The listing builds one solid part. Answer for the finished solid, in the listing's coordinates (mm). A direction names the side the tool comes from. Coordinates: 2 decimals unless noted, no trailing zeros. Write each loop counter-clockwise with the first axis right and the second up, starting at its lowest first coordinate (ties: lowest second). Pieces come first, ordered by that corner, then holes. Notation, with made-up numbers: M -8,-6 L 9,-6 A28 cw 9,22 Z; hole C 8,66.25 d3. An arc over 180 degrees is marked long. Answer as CSV lines item,"result". Start each with the question number.
```python
from build123d import *

# Parameters (mm, degrees)
F1_DEPTH       = 9.525
F2_D           = 5.5
F2_CBORE_D     = 9.75
F2_CBORE_DEPTH = 5
F3_R           = 5.08
F4_DEPTH       = 5
F5_D           = 5.5


# Not quite as in the source:
# - a feature names something its author has since deleted; it is built from what else it names


with BuildPart() as f1:
    # F0 (on Front) → F1 (new body)
    with BuildSketch(Plane.XZ):
        with BuildLine():
            Line((10, -40), (10, 0))
            ThreePointArc((10, 0), (7.0710678119, 7.0710678119), (0, 10))
            Line((0, 10), (-53.34, 10))
            ThreePointArc((-53.34, 10), (-62.826927837, 3.1619930765), (-59.3395200276, -8.0003599568))
            Line((-59.3395200276, -8.0003599568), (-5.9995200276, -48.0003599568))
            ThreePointArc((-5.9995200276, -48.0003599568), (4.4724042597, -48.9441377526), (10, -40))
        make_face()
        Polygon((-20.36, -4.1698729811), (-20.4062613559, -4.25), (-25.3137386441, -4.25), (-27.7674772881, 0), (-25.3137386441, 4.25), (-20.4062613559, 4.25), (-20.36, 4.1698729811), (-20.3137386441, 4.25), (-15.4062613559, 4.25), (-12.9525227119, 0), (-15.4062613559, -4.25), (-20.3137386441, -4.25), align=None, mode=Mode.SUBTRACT)
        Polygon((-25.3137386441, -4.25), (-20.4062613559, -4.25), (-20.36, -4.1698729811), (-22.7674772881, 0), (-20.36, 4.1698729811), (-20.4062613559, 4.25), (-25.3137386441, 4.25), (-27.7674772881, 0), align=None)
        Polygon((-17.9525227119, 0), (-20.36, -4.1698729811), (-20.3137386441, -4.25), (-15.4062613559, -4.25), (-12.9525227119, 0), (-15.4062613559, 4.25), (-20.3137386441, 4.25), (-20.36, 4.1698729811), align=None)
        Polygon((-22.7674772881, 0), (-20.36, -4.1698729811), (-17.9525227119, 0), (-20.36, 4.1698729811), align=None)
    extrude(amount=F1_DEPTH)

    # F2 (through all)
    with Locations(Plane(origin=(0, 0, 0), x_dir=(1, 0, 0), z_dir=(0, 1, 0))):
        with Locations((0, 0), (0, 40), (-53.34, 0)):
            CounterBoreHole(F2_D / 2, F2_CBORE_D / 2, F2_CBORE_DEPTH)

    # F3
    f3_edges = [f1.edges().sort_by_distance(p)[0] for p in [
        (-26.67, 0, 10),
    ]]
    fillet(f3_edges, radius=F3_R)

    # F0 (on Front) → F4 (cut)
    with BuildSketch(Plane.XZ):
        Polygon((-25.3137386441, -4.25), (-20.4062613559, -4.25), (-20.36, -4.1698729811), (-22.7674772881, 0), (-20.36, 4.1698729811), (-20.4062613559, 4.25), (-25.3137386441, 4.25), (-27.7674772881, 0), align=None)
        Polygon((-22.7674772881, 0), (-20.36, -4.1698729811), (-17.9525227119, 0), (-20.36, 4.1698729811), align=None)
        Polygon((-17.9525227119, 0), (-20.36, -4.1698729811), (-20.3137386441, -4.25), (-15.4062613559, -4.25), (-12.9525227119, 0), (-15.4062613559, 4.25), (-20.3137386441, 4.25), (-20.36, 4.1698729811), align=None)
    extrude(amount=F4_DEPTH, mode=Mode.SUBTRACT)

    # F5 (through all)
    with Locations(Plane(origin=(0, 0, 0), x_dir=(1, 0, 0), z_dir=(0, 1, 0))):
        with Locations((-22.86, 0)):
            Hole(F5_D / 2)


solid = f1.part
```
1) Which of the six approach directions +Z, -Z, +X, -X, +Y, -Y give full straight-line access (tool end or side, diameter ignored) to faces 4 (the face through (-26, -7, 10)), 5 (the face through (-18, -2, 4.25))?
2) The part is cut by section A-A (y = -8). Determine the outline of the cut face in (x, z).
3) Find the intervals of material crossed by line 1 (X direction, y = -3, z = 2); line 2 (X direction, y = -6, z = -8); line 3 (Z direction, x = -53.34, y = -5.9), in increasing order. Write a range as from..to.
4) Each of these flat-tipped pins is pushed along its axis until it touches: P1, Ø3.5, axis at x = 0, z = 0, coming from the -Y side; P2, Ø9, axis at x = 0, z = -40, coming from the +Y side; P3, Ø4, axis at x = -17, y = -2, coming from the +Z side; P4, Ø2.5, axis at x = -24, y = -2, coming from the -Z side. Where does it stop, or does it pass through?
5) For a pull along Z with two mould halves and no side action, classify faces 1 (the face through (-27.043, -1.449, 8.472)), 2 (the face through (-26.558, -2.465, -2.095)), 3 (the face through (-19, -9.525, -13)) as +Z half, -Z half, draft (parallel to the pull), parting line (faces both ways), or undercut.
Completed:
1,face 4,"+Z, +X, -X, +Y, -Y"
1,face 5,"+Y"
2,outline,"M -59.34,-8 L -6,-48 A10 ccw 10,-40 L 10,0 A10 ccw 0,10 L -53.34,10 A10 ccw Z; hole C -53.34,0 d5.5; hole C -22.86,0 d5.5; hole C 0,-40 d5.5; hole C 0,0 d5.5"
3,line 1,"-62.68..-57.79, -48.89..-26.61, -14.11..-4.45, 4.45..9.34"
3,line 2,"-59.34..10"
3,line 3,"-12.5..-2.75, 2.75..10"
4,P1,"through"
4,P2,"y = -5"
4,P3,"z = 9.88"
4,P4,"z = -34.55"
5,face 1,"+Z half"
5,face 2,"undercut"
5,face 3,"draft"
